Job drawing, mm, ordinate dimensions from the low corner. One solid piece. A direction names the side the tool comes from. Give positions to 0.01 mm unless a question says otherwise; leave off trailing zeros. Order: outer loops, then holes, each group sorted by start corner. A loop starts at its lowest first (then second) coordinate and runs counter-clockwise, first axis right, second up. Notation, with made-up numbers: M 53.5,-30.5 L 62.5,-30.5 A25 ccw 62.5,4.5 Z; hole C 28,35.5 d9. An arc over 180 degrees is marked long. Put each result on its own line as item: value. Start each with the question number.
1) Cut at A-A (z = 3.5). Write the cut outline in (x, y), and give its area (3 significant figures).
2) Two-plate mould, pull along X, no slides. Class the marked faces 1, 2 and 3: released by +X, released by -X, zero draft, split by the parting line, or undercut.
3) Tool access for the marked faces 4 and 5: list every direction of +Z, -Z, +X, -X, +Y, -Y with a clear straight run to the whole face (end or side of a thin tool).
4) Pin check, flat tips, straight feed: pin 1 (6 mm diameter, centred on y = 45.5, z = 7.5, fed in from +X); pin 2 (1 mm diameter, centred on y = 32, z = 7.5, fed in from -X); pin 3 (2 mm diameter, centred on x = 25, z = 4, fed in from +Y). Stop position of each tip, or through.
5) Drill centre lines: line 1 (X direction, y = 36, z = 3.25); line 2 (Y direction, x = 31.5, z = 9.25). Where is each one in solid material? Low to high. Write a range as [from, to].
6) Cut at C-C (y = 26). Write the cut outline in (x, z).
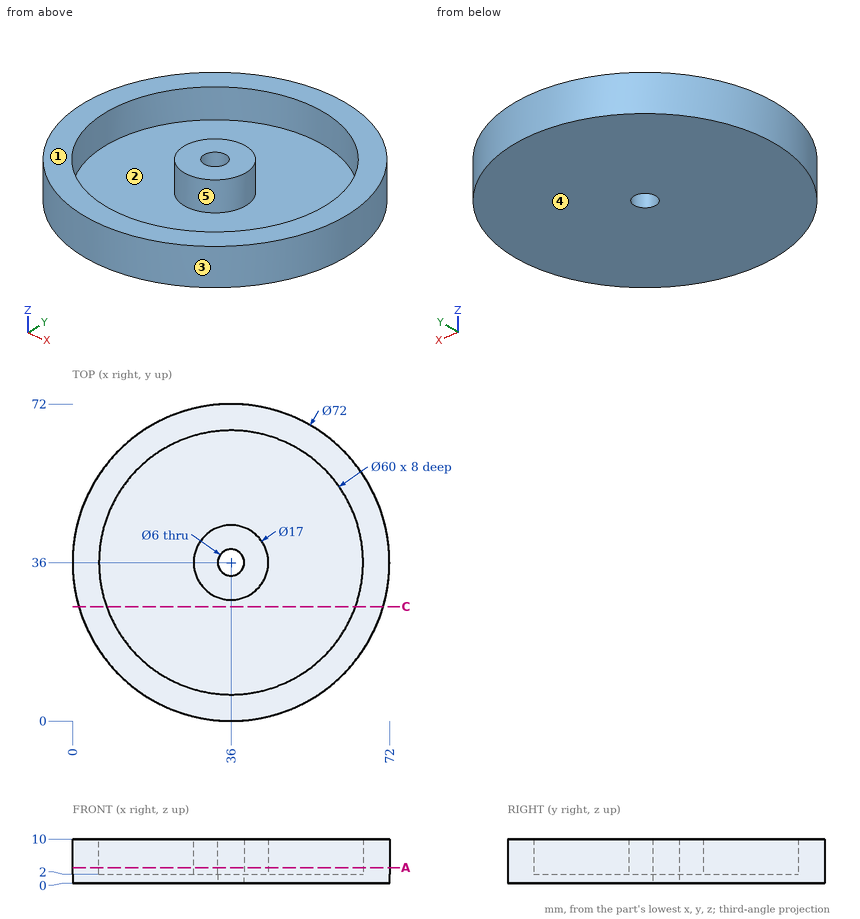
Solution:
1. outline: C 36,36 d72; C 36,36 d17; hole C 36,36 d60; hole C 36,36 d6
1. area: 1,440 mm²
2. face 1: zero draft
2. face 2: undercut
2. face 3: split by the parting line
3. face 4: -Z, +X, -X, +Y, -Y
3. face 5: +Z
4. pin 1: x = 71.41
4. pin 2: x = 0.17
4. pin 3: y = 70.58
5. line 1: [0, 6], [27.5, 33], [39, 44.5], [66, 72]
5. line 2: [0.28, 6.34], [28.79, 43.21], [65.66, 71.72]
6. outline: M 1.42,0 L 70.58,0 L 70.58,10 L 64.28,10 L 64.28,2 L 7.72,2 L 7.72,10 L 1.42,10 Z
